```python
from build123d import *

# Parameters (mm, degrees)
SKETCH1_R           = 1.1303
BOSS_EXTRUDE1_DEPTH = 82.55
CUT_EXTRUDE1_DEPTH  = 121.310224488


with BuildPart() as part:
    # Sketch1 → Boss-Extrude1 (new body)
    with BuildSketch(Plane(origin=(0, 0, 0), x_dir=(0, 0, -1), z_dir=(1, 0, 0))):
        with BuildLine():
            Line((-14.235037061, 4.6355), (4.911613569, 4.6355))
            Line((4.911613569, 4.6355), (4.911613569, 9.525))
            add(Edge.make_bspline(
                [(4.911613569, 9.525), (13.356859809, 9.525), (56.914542054, -6.988883897), (72.701512247, -37.41793147)],
                knots=[0, 0, 0, 0, 1, 1, 1, 1], degree=3))
            ThreePointArc((72.701512247, -37.41793147), (71.292110965, -42.742171877), (65.857227597, -41.849988788))
            add(Edge.make_bspline(
                [(-15.004369583, 0), (9.374116417, -8.321172008), (39.423381365, -8.534365891), (65.857227597, -41.849988788)],
                knots=[0, 0, 0, 0, 1, 1, 1, 1], degree=3))
            ThreePointArc((-15.004369583, 0), (-16.584490869, 2.643836713), (-14.235037061, 4.6355))
        make_face()
        Circle(SKETCH1_R, mode=Mode.SUBTRACT)
    extrude(amount=BOSS_EXTRUDE1_DEPTH)

    # Sketch2 → Cut-Extrude1 (cut, through all)
    with BuildSketch(Plane(origin=(0, 4.6355, 0), x_dir=(1, 0, 0), z_dir=(0, 1, 0))):
        Polygon((0, -4.661711746), (0, -18.489908959), (18.236274836, -18.489908959), align=None)
        Polygon((82.55, -4.661711746), (82.55, -18.489908959), (64.313725164, -18.489908959), align=None)
    extrude(amount=-CUT_EXTRUDE1_DEPTH, mode=Mode.SUBTRACT)


solid = part.part
```
Build history of the part. All positions in model axes, mm. A direction names the side the tool comes from. Coordinates: 2 decimals unless noted, no trailing zeros.
Item 1: Tool access for faces 1 (the cylindrical face through (40.697, -1.103, 0.245)), 2 (the flat face through (41, 4.636, 5)): list every direction of +Z, -Z, +X, -X, +Y, -Y with a clear straight run to the whole face (end or side of a thin tool).
Filled in:
face 1: +X, -X
face 2: +Z, +X, -X, +Y
Item 2: Drop flat-ended pins along their axis: pin 1 Ø5.5 at (x, y) = (51, 6.5) entering from +Z; pin 2 Ø10 at (x, z) = (43, -29) entering from +Y; pin 3 Ø1.4 at (y, z) = (0, 0) entering from +X; pin 4 Ø10 at (x, z) = (30.5, -49.5) entering from +Y. Give the stop position or say it passes through.
Filled in:
pin 1: stops at z = 16.09
pin 2: stops at y = 3.56
pin 3: passes through
pin 4: stops at y = -7.78
Item 3: Drill centre lines: L1, parallel to Y at x = 47, z = 0; L2, parallel to Z at x = 55.5, y = -14; L3, parallel to Y at x = 20, z = -64.5. Where is each one in solid material? Low to high.
Filled in:
L1: y = -4.29 to -1.13, 1.13 to 4.64
L2: z = -52.87 to -30.58
L3: y = -40.17 to -25.33
